Check sheet for the modelled part. Datum: model origin and axes. Units: mm. A direction names the side the tool comes from. Round coordinates to 2 decimals unless told otherwise and drop trailing zeros. Write each loop counter-clockwise with the first axis right and the second up, starting at its lowest first coordinate (ties: lowest second). Pieces come first, ordered by that corner, then holes. Notation, with made-up numbers: M 73,-5.5 L 113,-5.5 A25 ccw 113,22.5 Z; hole C 58,-38.75 d5. An arc over 180 degrees is marked long. One line per item, written item: value.
from build123d import *

# Parameters (mm, degrees)
SKETCH1_W           = 51
SKETCH1_H           = 25.68
BOSS_EXTRUDE1_DEPTH = 20
SKETCH3_W           = 45
SKETCH3_H           = 19.68
CUT_EXTRUDE1_DEPTH  = 17.5
CUT_EXTRUDE2_DEPTH  = 3
SKETCH5_W           = 10
SKETCH5_H           = 6
CUT_EXTRUDE3_DEPTH  = 3
SKETCH6_W           = 6
SKETCH6_H           = 6
SKETCH6_R           = 1.5
BOSS_EXTRUDE2_DEPTH = 20


with BuildPart() as part:
    # Sketch1 → Boss-Extrude1 (new body)
    with BuildSketch(Plane(origin=(0, 0, 0), x_dir=(1, 0, 0), z_dir=(0, 1, 0))):
        Rectangle(SKETCH1_W, SKETCH1_H)
    extrude(amount=BOSS_EXTRUDE1_DEPTH)

    # Sketch3 → Cut-Extrude1 (cut)
    with BuildSketch(Plane.XZ):
        Rectangle(SKETCH3_W, SKETCH3_H)
    extrude(amount=-CUT_EXTRUDE1_DEPTH, mode=Mode.SUBTRACT)

    # Sketch4 → Cut-Extrude2 (cut)
    with BuildSketch(Plane.XY.offset(12.84)):
        with BuildLine():
            Line((-17.5, 0), (17.5, 0))
            ThreePointArc((17.5, 0), (0, 17.5), (-17.5, 0))
        make_face()
    extrude(amount=-CUT_EXTRUDE2_DEPTH, mode=Mode.SUBTRACT)

    # Sketch5 → Cut-Extrude3 (cut)
    with BuildSketch(Plane(origin=(0, 0, -12.84), x_dir=(-1, 0, 0), z_dir=(0, 0, -1))):
        with Locations((-17, 3)):
            Rectangle(SKETCH5_W, SKETCH5_H)
    extrude(amount=-CUT_EXTRUDE3_DEPTH, mode=Mode.SUBTRACT)

    # Sketch6 → Boss-Extrude2 (add)
    with BuildSketch(Plane.XZ):
        with Locations((28.5, 0)):
            Rectangle(SKETCH6_W, SKETCH6_H)
        with Locations((28.5, 0)):
            Circle(SKETCH6_R, mode=Mode.SUBTRACT)
        with Locations((-28.5, 0)):
            Rectangle(SKETCH6_W, SKETCH6_H)
        with Locations((-28.5, 0)):
            Circle(SKETCH6_R, mode=Mode.SUBTRACT)
    extrude(amount=-BOSS_EXTRUDE2_DEPTH)


solid = part.part
Q1. Scan lines: line 1 (X direction, y = 13.25, z = -7.5); line 2 (Z direction, x = -28.5, y = 10.75); line 3 (Y direction, x = -20, z = 8.5). Record each from-to range of solid material in increasing order. Write a range as [from, to].
Completed:
line 1: [-25.5, -22.5], [22.5, 25.5]
line 2: [-3, -1.5], [1.5, 3]
line 3: [17.5, 20]
Q2. Depth check by flat-ended pin: P1, Ø2.5, axis at y = 2, z = -12, coming from the -X side; P2, Ø3, axis at x = -29, y = 13.5, coming from the -Z side; P3, Ø8, axis at x = 15.5, z = 4, coming from the -Y side. Enter the tip coordinate at first touch or a pass-through.
Completed:
P1: x = -25.5
P2: z = -3
P3: y = 17.5
Q3. Sectioned sample at A-A on y = 2.25. Enter the section's corners in (x, z), and give its area (3 significant figures).
Completed:
outline: M -31.5,-3 L -25.5,-3 L -25.5,-12.84 L 12,-12.84 L 12,-9.84 L -22.5,-9.84 L -22.5,9.84 L -17.35,9.84 L -17.35,12.84 L -25.5,12.84 L -25.5,3 L -31.5,3 Z; M 17.35,9.84 L 22.5,9.84 L 22.5,-9.84 L 22,-9.84 L 22,-12.84 L 25.5,-12.84 L 25.5,-3 L 31.5,-3 L 31.5,3 L 25.5,3 L 25.5,12.84 L 17.35,12.84 Z; hole C -28.5,0 d3; hole C 28.5,0 d3
area: 348 mm^2
Q4. Draft check along Z on faces 1 (the flat face through (0, 17.5, 0)), 2 (the flat face through (-16, 0, -11)), 3 (the flat face through (-29, 10, 3)). Enter one of: pulls with the +Z half, pulls with the -Z half, needs draft (parallel to the pull), parting line crosses it, or undercut.
Completed:
face 1: undercut
face 2: needs draft
face 3: pulls with the +Z half
Q5. Sectioned sample at B-B on z = 0. Enter the section's corners in (x, y), and give its area (4 significant figures).
Completed:
outline: M -31.5,0 L -30,0 L -30,20 L -31.5,20 Z; M -27,0 L -22.5,0 L -22.5,17.5 L 22.5,17.5 L 22.5,0 L 27,0 L 27,20 L -27,20 Z; M 30,0 L 31.5,0 L 31.5,20 L 30,20 Z
area: 352.5 mm^2
Q6. Sectioned sample at C-C on x = -28.5. Enter the section's corners in (y, z), and give its area (3 significant figures).
Completed:
outline: M 0,-3 L 20,-3 L 20,-1.5 L 0,-1.5 Z; M 0,1.5 L 20,1.5 L 20,3 L 0,3 Z
area: 60.0 mm^2
Q7. Access from +Z, -Z, +X, -X, +Y, -Y to the whole of each face (thin tool, end or side, straight path). Record for faces 4 (the cylindrical face through (0.385, 17.496, 11.361)), 5 (the flat face through (12, 3, -11)), 6 (the flat face through (25.5, 10, 8)), 7 (the flat face through (-29, 10, -3)).
Completed:
face 4: +Z, -Y
face 5: +Z, -Z, -Y
face 6: +Z, +X, +Y, -Y
face 7: -Z, -X, +Y, -Y
Q8. Sectioned sample at D-D on z = 4. Enter the section's corners in (x, y).
Completed:
outline: M -25.5,0 L -22.5,0 L -22.5,17.5 L 22.5,17.5 L 22.5,0 L 25.5,0 L 25.5,20 L -25.5,20 Z
